from build123d import *

# Parameters (mm, degrees)
SKETCH_1_W          = 100
SKETCH_1_H          = 80
EXTRUDE_1_DEPTH     = 39
SKETCH_5_R          = 3
EXTRUDE_3_DEPTH     = 10
CUT_EXTRUDE_1_DEPTH = 1000
SKETCH_9_W          = 20
SKETCH_9_H          = 6.479518585
SKETCH_9_H_2        = 3
SKETCH_9_H_3        = 8.519653391
SKETCH_9_H_4        = 11.10220699
SKETCH_9_H_5        = 8.801039891
CUT_EXTRUDE_3_DEPTH = 36
SKETCH_10_R         = 2.5
CUT_EXTRUDE_4_DEPTH = 36


with BuildPart() as part:
    # 草图1 → 凸台-拉伸1 (new body)
    with BuildSketch(Plane(origin=(0, 0, 0), x_dir=(1, 0, 0), z_dir=(0, 1, 0))):
        with Locations((50, -40)):
            Rectangle(SKETCH_1_W, SKETCH_1_H)
    extrude(amount=EXTRUDE_1_DEPTH)

    # 草图5 → 凸台-拉伸3 (add)
    with BuildSketch(Plane(origin=(100, 0, 0), x_dir=(0, 0, -1), z_dir=(1, 0, 0))):
        with Locations(Location((-50.5, 6, 0), (0, 0, 180))):
            Circle(SKETCH_5_R)
        with Locations(Location((-43.5, 6, 0), (0, 0, 180))):
            Circle(SKETCH_5_R)
        with Locations(Location((-36.5, 6, 0), (0, 0, 180))):
            Circle(SKETCH_5_R)
        with Locations(Location((-29.5, 6, 0), (0, 0, 180))):
            Circle(SKETCH_5_R)
    extrude(amount=EXTRUDE_3_DEPTH)

    # 草图8 → 切除-拉伸1 (cut)
    with BuildSketch(Plane(origin=(100, 0, 0), x_dir=(0, 0, -1), z_dir=(1, 0, 0))):
        Polygon((-78, 3), (-75, 39), (-80, 39), (-80, 3), align=None)
        Polygon((0, 3), (0, 39), (-5, 39), (-2, 3), align=None)
    extrude(amount=-CUT_EXTRUDE_1_DEPTH, mode=Mode.SUBTRACT)

    # 草图9 → 切除-拉伸3 (cut)
    with BuildSketch(Plane(origin=(0, 39, 0), x_dir=(1, 0, 0), z_dir=(0, 1, 0))):
        with Locations((25, -1.760240707)):
            Rectangle(SKETCH_9_W, SKETCH_9_H)
        with Locations((25, -6.5)):
            Rectangle(SKETCH_9_W, SKETCH_9_H_2)
        with Locations((75, -0.740173304)):
            Rectangle(SKETCH_9_W, SKETCH_9_H_3)
        with Locations((75, -6.5)):
            Rectangle(SKETCH_9_W, SKETCH_9_H_2)
        with Locations((75, -80.551103495)):
            Rectangle(SKETCH_9_W, SKETCH_9_H_4)
        with Locations((75, -73.5)):
            Rectangle(SKETCH_9_W, SKETCH_9_H_2)
        with Locations((25, -79.400519946)):
            Rectangle(SKETCH_9_W, SKETCH_9_H_5)
        with Locations((25, -73.5)):
            Rectangle(SKETCH_9_W, SKETCH_9_H_2)
    extrude(amount=-CUT_EXTRUDE_3_DEPTH, mode=Mode.SUBTRACT)

    # 草图10 → 切除-拉伸4 (cut)
    with BuildSketch(Plane(origin=(0, 3, 0), x_dir=(1, 0, 0), z_dir=(0, 1, 0))):
        with Locations(Location((25, -4, 0), (0, 0, 270))):
            Circle(SKETCH_10_R)
        with Locations(Location((25.358741031, -75.748206295, 0), (0, 0, 270))):
            Circle(SKETCH_10_R)
        with Locations(Location((75, -4, 0), (0, 0, 270))):
            Circle(SKETCH_10_R)
        with Locations(Location((74.641258969, -75.748206295, 0), (0, 0, 270))):
            Circle(SKETCH_10_R)
    extrude(amount=-CUT_EXTRUDE_4_DEPTH, mode=Mode.SUBTRACT)


solid = part.part
Input: part model. Units: mm. Frame: model coordinates. A direction names the side the tool comes from. Coordinates: 2 decimals unless noted, no trailing zeros. Loops run counter-clockwise (first coordinate to the right, second up) from the corner with the lowest first, then second, coordinate; pieces in that order, holes last. Notation, with made-up numbers: (78, -32) -> (87, -32) arc R36 cw to (87, 6) -> close; hole circle Ø5 at (48, 21). An arc over 180 degrees is marked (long way). Write item = value, one per line. Start each with the question number.
Item 1: Cut plane B-B, the plane x = 91.5. Return loops of the section in (y, z), plus the area to 3 significant figures.
Item 2: Material intervals for line 1 (X direction, y = 29, z = 7.5); line 2 (X direction, y = 1.55, z = 4); line 3 (X direction, y = 24, z = 62), sorted ascending.
Item 3: Mould query, pull axis Z, two halves, no side actions, for faces 4 (the face through (75, 21, 8)), 5 (the face through (25, 21, 72)), 6 (the face through (72.2, 1.52, 75.21)), 7 (the face through (65, 21, 6)). Classes: pulls with the +Z half, pulls with the -Z half, needs draft (parallel to the pull), parting line crosses it, or undercut.
Item 4: Reachability of faces 1 (the face through (35, 21, 6)), 2 (the face through (15, 21, 74)), 3 (the face through (104.9, 5.9, 47.5)) from +Z, -Z, +X, -X, +Y, -Y: full face, straight path, thin tool, end or side. Return the list, or none.
Item 5: Cut plane D-D, the plane x = 102.5. Return loops of the section in (y, z), plus the area to 3 significant figures.
Item 6: Cut plane C-C, the plane z = 36.5. Return loops of the section in (x, y), plus the area to 3 significant figures.
Item 7: Cut plane A-A, the plane y = 24. Return loops of the section in (x, z), plus the area to 3 significant figures.
Item 8: First-contact query: P1, Ø6.5, axis at y = 24.5, z = 74, coming from the +X side; P2, Ø8, axis at x = 27.5, y = 31, coming from the +Z side; P3, Ø16, axis at x = 70.5, y = 12, coming from the +Z side; P4, Ø6, axis at x = 74.64, z = 75.75, coming from the -Y side. Flat tips, straight axial feed; report the tip coordinate or a pass-through.
Ans:
q1.outline = (0, 0) -> (3, 0) -> (3, 2) -> (39, 5) -> (39, 75) -> (3, 78) -> (3, 80) -> (0, 80) -> close
q1.area = 2,870 mm²
q2.line_1 = 0 to 15, 35 to 65, 85 to 100
q2.line_2 = 0 to 22.5, 27.5 to 72.5, 77.5 to 100
q2.line_3 = 0 to 100
q3.face_4 = pulls with the -Z half
q3.face_5 = pulls with the +Z half
q3.face_6 = undercut
q3.face_7 = needs draft
q4.face_1 = -Z, +Y
q4.face_2 = +Z, +Y
q4.face_3 = +X
q5.outline = circle Ø6 at (6, 29.5); circle Ø6 at (6, 36.5); circle Ø6 at (6, 43.5); circle Ø6 at (6, 50.5)
q5.area = 113 mm²
q6.outline = (0, 0) -> (100, 0) -> (100, 3) -> (110, 3) -> (110, 9) -> (100, 9) -> (100, 39) -> (0, 39) -> close
q6.area = 3,960 mm²
q7.outline = (0, 3.75) -> (15, 3.75) -> (15, 8) -> (35, 8) -> (35, 3.75) -> (65, 3.75) -> (65, 8) -> (85, 8) -> (85, 3.75) -> (100, 3.75) -> (100, 76.25) -> (85, 76.25) -> (85, 72) -> (65, 72) -> (65, 76.25) -> (35, 76.25) -> (35, 72) -> (15, 72) -> (15, 76.25) -> (0, 76.25) -> close
q7.area = 6,910 mm²
q8.P1 = 100
q8.P2 = 72
q8.P3 = 77.73
q8.P4 = 0
